Build history of the part. All positions in model axes, mm. A direction names the side the tool comes from. Give positions to 0.01 mm unless a question says otherwise; leave off trailing zeros.
from build123d import *

# Parameters (mm, degrees)
F0_R      = 12.7
F1_DEPTH  = 38.1
F3_D      = 11.90752
F3_DEPTH  = 15.4214285714
F3_TIP    = 3.5773799191
F5_D      = 6.35
F7_D      = 5.842
F7_DEPTH  = 25.4
F7_TIP    = 1.7551138682
F11_SIZE2 = 3.175
F11_SIZE  = 21.59
F13_DEPTH = 12.7


with BuildPart() as f1:
    # F0 (on Front) → F1 (new body)
    with BuildSketch(Plane.XZ):
        Circle(F0_R)
    extrude(amount=F1_DEPTH)

    # F3
    with Locations(Plane(origin=(0, 0, 0), x_dir=(-1, 0, 0), z_dir=(0, 1, 0))):
        with Locations((0, 0)):
            Hole(F3_D / 2, depth=F3_DEPTH)
            with Locations((0, 0, -(F3_DEPTH + F3_TIP / 2))):  # 118° drill point
                Cone(0, F3_D / 2, F3_TIP, mode=Mode.SUBTRACT)

    # F5 (through all)
    with Locations(Plane.XZ.offset(38.1)):
        with Locations((0, 0)):
            Hole(F5_D / 2)

    # F7
    with Locations(Plane.XZ.offset(38.1)):
        with Locations((0, 7.9375), (-5.6126600757, 5.6126600757), (-7.9375, 0), (-5.6126600757, -5.6126600757), (0, -7.9375), (5.6126600757, -5.6126600757), (7.9375, 0), (5.6126600757, 5.6126600757)):
            Hole(F7_D / 2, depth=F7_DEPTH)
            with Locations((0, 0, -(F7_DEPTH + F7_TIP / 2))):  # 118° drill point
                Cone(0, F7_D / 2, F7_TIP, mode=Mode.SUBTRACT)

    # F11
    f11_edges = [f1.edges().sort_by_distance(p)[0] for p in [
        (-12.7, 0, 0),
    ]]
    f11_side = f1.faces().sort_by_distance((-12.7, -19.05, 0))[0]
    chamfer(f11_edges, length=F11_SIZE, length2=F11_SIZE2, reference=f11_side)

    # F12 (on Right) → F13 (cut, symmetric)
    with BuildSketch(Plane.YZ):
        Polygon((-43.4335693717, -3.8883644156), (-38.1641536951, -4.8853410408), (-19.5609088987, 14.8634454235), (-39.1272343695, 17.5419766456), align=None)
    extrude(amount=F13_DEPTH, both=True, mode=Mode.SUBTRACT)


solid = f1.part
1. Drop flat-ended pins along their axis: pin 1 (9.5 mm diameter, centred on x = 5.61, z = -5.61, fed in from -Y); pin 2 (3.5 mm diameter, centred on x = -7.94, z = 0, fed in from -Y); pin 3 (3 mm diameter, centred on y = -31.5, z = -6, fed in from +X); pin 4 (6.5 mm diameter, centred on x = 0, z = 7.94, fed in from -Y). Give the stop position or say it passes through.
2. Saw through at A-A on x = -1. Count the separate pieces of the cut face and the enclosed holes in it, plus the area to 3 significant figures.
3. 3-axis set-ups, long thin cutter, end or side, ignore diameter. For faces 1 (the face through (0.63, -25.22, -10.79)), 2 (the face through (5.5, -6.11, -2.28)), 3 (the face through (-0.2, -38.1, -11.3)): which of +Z, -Z, +X, -X, +Y, -Y reach the whole face in a straight line?
4. Drill centre lines: line 1 along Z through (x, y) = (4, -19); line 2 along Z through (x, y) = (-7.5, -23.5); line 3 along X through (y, z) = (-35, -6.75). Where is each one in solid material? Low to high.
5. Mould opens along X. For faces 4 (the face through (-0.1, 0, -6.2)), 5 (the face through (-9.29, -24.37, -2.59)), 6 (the face through (10.24, -8.24, 3.23)) say: pulls with the +X half, pulls with the -X half, needs draft (parallel to the pull), parting line crosses it, or undercut.
Outcome:
1. pin 1: stops at y = -38.1
1. pin 2: stops at y = -12
1. pin 3: stops at x = 11.88
1. pin 4: stops at y = -29.14
2. separate pieces: 4
2. enclosed holes: 0
2. area: 241 mm2
3. face 1: -Y
3. face 2: +Y
3. face 3: +Z, -Z, +X, -X, -Y
4. line 1: z = -11.65 to -8.05, -3.18 to 3.18, 8.05 to 11.65
4. line 2: z = -10.25 to -7.84, -3.38 to -2.89, 2.89 to 3.38, 7.84 to 10.25
4. line 3: x = -10.76 to -8.3, -2.92 to -2.67, 2.67 to 2.92, 8.3 to 10.76
5. face 4: needs draft
5. face 5: undercut
5. face 6: parting line crosses it
